```python
from build123d import *

# Parameters (mm, degrees)
F1_DEPTH = 5.08
F2_R     = 2.53999
F3_R     = 1.905
F4_DEPTH = 25.4
F5_R     = 1.905
F6_DEPTH = 5.08


# Not quite as in the source:
# - a fillet or chamfer is up to 0.001 mm smaller than in the source, because OpenCascade refuses the exact size


with BuildPart() as f1:
    # F0 (on Top) → F1 (new body)
    with BuildSketch(Plane.XY):
        Polygon((10.16, 0), (0, 0), (0, -5.08), (10.16, -5.08), (10.16, -3.556), (16.51, -3.556), (16.51, -1.524), (10.16, -1.524), align=None)
    extrude(amount=F1_DEPTH)

    # F2 (radius 2.54 in the source; OpenCascade refuses exactly that, so slightly less here)
    f2_edges = [f1.edges().sort_by_distance(p)[0] for p in [
        (16.51, -2.54, 5.08),
        (16.51, -2.54, 0),
        (0, -2.54, 5.08),
        (0, -2.54, 0),
    ]]
    fillet(f2_edges, radius=F2_R)

    # F3 (on face) → F4 (cut)
    with BuildSketch(Plane(origin=(0, -1.524, 0), x_dir=(-1, 0, 0), z_dir=(0, 1, 0))):
        with Locations((-13.97, 2.54)):
            Circle(F3_R)
    extrude(amount=-F4_DEPTH, mode=Mode.SUBTRACT)

    # F5 (on face) → F6 (cut)
    with BuildSketch(Plane(origin=(0, 0, 0), x_dir=(-1, 0, 0), z_dir=(0, 1, 0))):
        with Locations((-2.54, 2.54)):
            Circle(F5_R)
    extrude(amount=-F6_DEPTH, mode=Mode.SUBTRACT)


solid = f1.part
```
CAD build for the part. Positions are in the model's coordinates, mm. A direction names the side the tool comes from. Round coordinates to 2 decimals unless told otherwise and drop trailing zeros. Write each loop counter-clockwise with the first axis right and the second up, starting at its lowest first coordinate (ties: lowest second). Pieces come first, ordered by that corner, then holes. Notation, with made-up numbers: (30.5, -37.75) - (78.5, -37.75) arc R28 cw to (78.5, -4.75) - close; hole circle Ø11 at (73.25, 62.25). An arc over 180 degrees is marked (long way). Return JSON: item names as keys, results as strings. Group by question number.
Item 1: Band-saw the part on B-B on z = 2.1. List the corners of the cut face in (x, y), plus the area to 3 significant figures.
Item 2: Band-saw the part on A-A on x = 2. List the corners of the cut face in (y, z).
Item 3: Band-saw the part on D-D on z = 3.2. List the corners of the cut face in (x, y), plus the area to 3 significant figures.
Item 4: 3-axis set-ups, long thin cutter, end or side, ignore diameter. For faces 1 (the face through (10.16, -4, 3)), 2 (the face through (10.16, -1, 3)), 3 (the face through (15.8, -2.5, 4.3)): which of +Z, -Z, +X, -X, +Y, -Y reach the whole face in a straight line?
Item 5: Band-saw the part on C-C on x = 12.25. List the corners of the cut face in (y, z).
Item 6: Mould opens along Z. For faces 4 (the face through (6, 0, 3)), 5 (the face through (12.153, -2.526, 3.112)), 6 (the face through (15.786, -2.526, 0.764)) say: +Z half, -Z half, draft (parallel to the pull), parting line (faces both ways), or undercut.
Item 7: Flat gauge pins, fed straight in: pin 1 Ø0.5 at (y, z) = (-1, 2.5) entering from +X; pin 2 Ø1 at (y, z) = (-3.5, 3) entering from -X; pin 3 Ø3 at (x, z) = (13.97, 2.54) entering from -Y. Where does each tip first touch, or does it go through?
Item 8: Probe probe 1 along Z at (x, y) = (13.97, -2) (3 decimals); probe 2 along X at (y, z) = (-1.95, 1.1); probe 3 along X at (y, z) = (-2.7, 3). List the from-to ranges inside material, lowest first.
Resolved:
{
 "1": {"outline": "(0.04, -5.08) - (0.69, -5.08) - (0.69, 0) - (0.04, 0) - close; (4.39, -5.08) - (10.16, -5.08) - (10.16, -3.56) - (12.12, -3.56) - (12.12, -1.52) - (10.16, -1.52) - (10.16, 0) - (4.39, 0) - close; (15.82, -3.56) - (16.47, -3.56) - (16.47, -1.52) - (15.82, -1.52) - close", "area": "37.9 mm²"},
 "2": {"outline": "(-5.08, 0.06) - (0, 0.06) - (0, 0.71) - (-5.08, 0.71) - close; (-5.08, 4.37) - (0, 4.37) - (0, 5.02) - (-5.08, 5.02) - close"},
 "3": {"outline": "(0.09, -5.08) - (0.75, -5.08) - (0.75, 0) - (0.09, 0) - close; (4.33, -5.08) - (10.16, -5.08) - (10.16, -3.56) - (12.18, -3.56) - (12.18, -1.52) - (10.16, -1.52) - (10.16, 0) - (4.33, 0) - close; (15.76, -3.56) - (16.42, -3.56) - (16.42, -1.52) - (15.76, -1.52) - close", "area": "38.5 mm²"},
 "4": {"face 1": "+Z, -Z, +X, -Y", "face 2": "+Z, -Z, +X, +Y", "face 3": "+Z, +X, +Y, -Y"},
 "5": {"outline": "(-3.56, 0) - (-1.52, 0) - (-1.52, 1.72) - (-3.56, 1.72) - close; (-3.56, 3.36) - (-1.52, 3.36) - (-1.52, 5.08) - (-3.56, 5.08) - close"},
 "6": {"face 4": "draft", "face 5": "undercut", "face 6": "-Z half"},
 "7": {"pin 1": "stops at x = 10.16", "pin 2": "stops at x = 0", "pin 3": "passes through"},
 "8": {"probe 1": "z = 0 to 0.635, 4.445 to 5.08", "probe 2": "x = 0.45 to 1.29, 3.79 to 12.72, 15.22 to 16.06", "probe 3": "x = 0.04 to 0.69, 4.39 to 12.12, 15.82 to 16.47"}
}
